Can you work these out from the model? Positions are in its coordinate system, mm. Give positions to 0.01 mm unless a question says otherwise; leave off trailing zeros. Order: outer loops, then holes, each group sorted by start corner. A loop starts at its lowest first (then second) coordinate and runs counter-clockwise, first axis right, second up. Notation, with made-up numbers: (31.5, 8.25) - (64.5, 8.25) arc R29 cw to (64.5, 37.25) - close; hole circle Ø11 at (-8.5, 58.5). An arc over 180 degrees is marked (long way). Return JSON: item names as keys, results as strings.
```python
from build123d import *

# Parameters (mm, degrees)
ESQUISSE1_W             = 140
ESQUISSE1_H             = 100
BOSS_EXTRU_1_DEPTH      = 2
ESQUISSE2_W             = 55
ESQUISSE2_H             = 66
ENL_V_MAT_EXTRU_1_DEPTH = 2
ESQUISSE3_W             = 78
ESQUISSE3_H             = 10
ESQUISSE3_W_2           = 2
ENL_V_MAT_EXTRU_2_DEPTH = 3


with BuildPart() as part:
    # Esquisse1 → Boss.-Extru.1 (new body)
    with BuildSketch(Plane.XY):
        with Locations((70, 50)):
            Rectangle(ESQUISSE1_W, ESQUISSE1_H)
    extrude(amount=BOSS_EXTRU_1_DEPTH)

    # Esquisse2 → Enlèv. mat.-Extru.1 (cut)
    with BuildSketch(Plane.XY.offset(2)):
        with Locations((107.5, 50)):
            Rectangle(ESQUISSE2_W, ESQUISSE2_H)
    extrude(amount=-ENL_V_MAT_EXTRU_1_DEPTH, mode=Mode.SUBTRACT)

    # Esquisse3 → Enlèv. mat.-Extru.2 (cut)
    with BuildSketch(Plane.XY.offset(2)):
        with Locations((39, 52)):
            Rectangle(ESQUISSE3_W, ESQUISSE3_H)
        with Locations((79, 52)):
            Rectangle(ESQUISSE3_W_2, ESQUISSE3_H)
    extrude(amount=-ENL_V_MAT_EXTRU_2_DEPTH, mode=Mode.SUBTRACT)


solid = part.part
```
1. Suppose I cut it at B-B (y = 31.5). List the corners of the cut face in (x, z) for me, plus the area to 3 significant figures.
Checks:
{"outline": "(0, 0) - (80, 0) - (80, 2) - (0, 2) - close; (135, 0) - (140, 0) - (140, 2) - (135, 2) - close", "area": "170 mm^2"}
2. Suppose I cut it at A-A (x = 66.5). List the corners of the cut face in (y, z) for me.
Checks:
{"outline": "(0, 0) - (47, 0) - (47, 2) - (0, 2) - close; (57, 0) - (100, 0) - (100, 2) - (57, 2) - close"}
3. Suppose I cut it at C-C (z = 1.55). List the corners of the cut face in (x, y) for me, plus the area to 3 significant figures.
Checks:
{"outline": "(0, 0) - (140, 0) - (140, 100) - (0, 100) - (0, 57) - (80, 57) - (80, 83) - (135, 83) - (135, 17) - (80, 17) - (80, 47) - (0, 47) - close", "area": "9,570 mm^2"}
4. If I drill on L1, parallel to Y at x = 98.5, z = 1.05; L2, parallel to X at y = 65.5, z = 1.9; L3, parallel to Y at x = 51.5, z = 1.9, over which ranges is the centre line in solid material (lowest first)? Write a range as [from, to].
Checks:
{"L1": "[0, 17], [83, 100]", "L2": "[0, 80], [135, 140]", "L3": "[0, 47], [57, 100]"}
